The listing builds one solid part. Answer for the finished solid, in the listing's coordinates (mm). A direction names the side the tool comes from. Coordinates: 2 decimals unless noted, no trailing zeros. Order: outer loops, then holes, each group sorted by start corner. A loop starts at its lowest first (then second) coordinate and runs counter-clockwise, first axis right, second up.
from build123d import *

# Parameters (mm, degrees)
F0_R     = 225
F0_R_2   = 60.5
F1_DEPTH = 15
F2_R     = 225
F2_R_2   = 60.5
F3_DEPTH = 20


with BuildPart() as f1:
    # F0 (on Right) → F1 (new body, symmetric)
    with BuildSketch(Plane.YZ):
        with BuildLine():
            Line((-726.5, 100), (-726.5, 0))
            Line((-726.5, 0), (726.5, 0))
            ThreePointArc((726.5, 0), (976.5, 250), (726.5, 500))
            Line((726.5, 500), (273.5, 500))
            Line((273.5, 500), (-726.5, 100))
        make_face()
        with Locations((726.5, 250)):
            Circle(F0_R, mode=Mode.SUBTRACT)
        with Locations((726.5, 250)):
            Circle(F0_R)
        with Locations((726.5, 250)):
            Circle(F0_R_2, mode=Mode.SUBTRACT)
    extrude(amount=F1_DEPTH, both=True)

    # F2 (on face) → F3 (join)
    with BuildSketch(Plane(origin=(-15, 0, 0), x_dir=(0, -1, 0), z_dir=(-1, 0, 0))):
        with Locations((-726.5, 250)):
            Circle(F2_R)
        with Locations((-726.5, 250)):
            Circle(F2_R_2, mode=Mode.SUBTRACT)
    extrude(amount=F3_DEPTH)

    # F4: F1 across plane


with BuildPart() as f1_1:
    add(f1.part)
    add(f1.part.mirror(Plane.YZ))


solid = f1_1.part
1) Section B-B (x = 3) is taken. Give the vertices of the cut face in (y, z).
2) Consider L1, parallel to Z at x = 1, y = 726; L2, parallel to Z at x = 25.25, y = 726.5; L3, parallel to X at y = 281, z = 360.5. Determine where each line is inside the solid, lowest interval first.
3) Section C-C (y = -275) is taken. Give the vertices of the cut face in (x, z), then the cut area to 3 significant figures.
4) Section A-A (z = 250) is taken. Give the vertices of the cut face in (x, y).
5) Each of these flat-tipped pins is pushed along its axis until it touches: P1, Ø6, axis at x = -11.5, z = 277, coming from the +Y side; P2, Ø10, axis at x = -26, z = 363, coming from the +Y side; P3, Ø6, axis at x = -3.5, y = -79.5, coming from the +Z side. Where does it stop, or does it pass through?
6) A tool of negligible diameter and unlimited length cuts with its end or side. For faces 1 (the face through (24.86, 755.791, 473.085)), 2 (the face through (0.21, 976.44, 244.5)), 3 (the face through (-24.86, 755.791, 473.085)), from which of +Z, -Z, +X, -X, +Y, -Y can it reach the whole face along a straight path? Write none if from no direction.
7) Section D-D (z = 359) is taken. Give the vertices of the cut face in (x, y).
Filled sheet:
1. outline: (-726.5, 0) - (726.5, 0) arc R250 ccw to (726.5, 500) - (273.5, 500) - (-726.5, 100) - close; hole circle Ø121 at (726.5, 250)
2. L1: z = 0 to 189.5, 310.5 to 500
2. L2: z = 25 to 189.5, 310.5 to 475
2. L3: x = -15 to 15
3. outline: (-15, 0) - (15, 0) - (15, 280.6) - (-15, 280.6) - close
3. area: 8,420 mm2
4. outline: (-35, 501.5) - (-15, 501.5) - (-15, -351.5) - (15, -351.5) - (15, 501.5) - (35, 501.5) - (35, 666) - (-35, 666) - close; (-35, 787) - (35, 787) - (35, 951.5) - (15, 951.5) - (15, 976.5) - (-15, 976.5) - (-15, 951.5) - (-35, 951.5) - close
5. P1: stops at y = 975.35
5. P2: stops at y = 923.89
5. P3: stops at z = 360
6. face 1: +X
6. face 2: +X, -X, +Y
6. face 3: -X
7. outline: (-35, 529.67) - (-15, 529.67) - (-15, -79) - (15, -79) - (15, 529.67) - (35, 529.67) - (35, 923.33) - (15, 923.33) - (15, 951.49) - (-15, 951.49) - (-15, 923.33) - (-35, 923.33) - close
